Work out the finished part from the listing and answer in its coordinate system (mm). Coordinates: 2 decimals unless noted, no trailing zeros. Order: outer loops, then holes, each group sorted by start corner. A loop starts at its lowest first (then second) coordinate and runs counter-clockwise, first axis right, second up.
1. The part is cut by section A-A, the plane x = -12.5. Give the vertices of the cut face in (y, z).
2. A flat-ended cylindrical pin translates along its axis: pin 1 Ø2 at (x, y) = (12.68, -25.38) entering from -Z. Find the tip coordinate at first contact, or state that the pin passes through.
3. The part is cut by section B-B, the plane z = 1.3. Give the vertices of the cut face in (x, y).
4. Find the intervals of material crossed by probe 1 along Y at (x, z) = (12.5, 0.75); probe 2 along Y at (x, z) = (11.5, 2.4); probe 3 along X at (y, z) = (-26.5, 0.1), in increasing order.
5. Determine the mould class of faces 1 (the flat face through (1, -10, 3)), 2 (the cylindrical face through (-9.594, 5.168, 1.479)), 3 (the flat face through (5, 14.623, 1)), 4 (the flat face through (6, -35.377, 1)) for opening direction Y: +Y half, -Y half, draft (parallel to the pull), parting line (faces both ways), or undercut.
6. The part is cut by section C-C, the plane y = 5.5. Give the vertices of the cut face in (x, z), then the cut area to 3 significant figures.
```python
from build123d import *

# Parameters (mm, degrees)
SKETCH1_R           = 1.814467449
SKETCH1_R_2         = 1.995778983
SKETCH1_R_3         = 2.141873052
SKETCH1_R_4         = 1.87301365
BOSS_EXTRUDE1_DEPTH = 3


with BuildPart() as part:
    # Sketch1 → Boss-Extrude1 (new body)
    with BuildSketch(Plane.XY):
        with BuildLine():
            Line((-13.324675325, 14.623376623), (24.675324675, 14.623376623))
            Line((24.675324675, 14.623376623), (24.675324675, -35.376623377))
            Line((24.675324675, -35.376623377), (-13.324675325, -35.376623377))
            ThreePointArc((-13.324675325, -35.376623377), (-20.395743137, -32.447691188), (-23.324675325, -25.376623377))
            Line((-23.324675325, -25.376623377), (-23.324675325, 4.623376623))
            ThreePointArc((-23.324675325, 4.623376623), (-20.395743137, 11.694444435), (-13.324675325, 14.623376623))
        make_face()
        with Locations((-11.324675325, 4.623376623)):
            Circle(SKETCH1_R, mode=Mode.SUBTRACT)
        with Locations((12.675324675, 4.623376623)):
            Circle(SKETCH1_R_2, mode=Mode.SUBTRACT)
        with Locations((-11.324675325, -25.376623377)):
            Circle(SKETCH1_R_3, mode=Mode.SUBTRACT)
        with Locations((12.675324675, -25.376623377)):
            Circle(SKETCH1_R_4, mode=Mode.SUBTRACT)
    extrude(amount=BOSS_EXTRUDE1_DEPTH)


solid = part.part
```
Geometry says:
1. outline: (-35.38, 0) - (-27.17, 0) - (-27.17, 3) - (-35.38, 3) - close; (-23.59, 0) - (3.24, 0) - (3.24, 3) - (-23.59, 3) - close; (6.01, 0) - (14.62, 0) - (14.62, 3) - (6.01, 3) - close
2. pin 1: passes through
3. outline: (-23.32, -25.38) arc R10 ccw to (-13.32, -35.38) - (24.68, -35.38) - (24.68, 14.62) - (-13.32, 14.62) arc R10 ccw to (-23.32, 4.62) - close; hole circle Ø4.28 at (-11.32, -25.38); hole circle Ø3.63 at (-11.32, 4.62); hole circle Ø3.99 at (12.68, 4.62); hole circle Ø3.75 at (12.68, -25.38)
4. probe 1: y = -35.38 to -27.24, -23.51 to 2.64, 6.61 to 14.62
4. probe 2: y = -35.38 to -26.83, -23.92 to 3.01, 6.24 to 14.62
4. probe 3: x = -23.26 to -13.15, -9.5 to 11.18, 14.17 to 24.68
5. face 1: draft
5. face 2: undercut
5. face 3: +Y half
5. face 4: -Y half
6. outline: (-23.29, 0) - (-12.91, 0) - (-12.91, 3) - (-23.29, 3) - close; (-9.74, 0) - (10.88, 0) - (10.88, 3) - (-9.74, 3) - close; (14.47, 0) - (24.68, 0) - (24.68, 3) - (14.47, 3) - close
6. area: 124 mm2
